Source: CAD feature listing. Evaluate the final solid. Frame: model axes, mm. Round coordinates to 2 decimals unless told otherwise and drop trailing zeros. Loops run counter-clockwise (first coordinate to the right, second up) from the corner with the lowest first, then second, coordinate; pieces in that order, holes last. Notation, with made-up numbers: (-22.75, -38) -> (6.25, -38) arc R35 cw to (6.25, -6) -> close; hole circle Ø9 at (-40, 11.25). An arc over 180 degrees is marked (long way). Write item = value, one per line.
from build123d import *

# Parameters (mm, degrees)
F1_DEPTH = 6.35
F2_R     = 2
F3_DEPTH = 20000
F4_R     = 7.5
F5_DEPTH = 55.3


with BuildPart() as f1:
    # F0 (on Top) → F1 (new body)
    with BuildSketch(Plane.XY):
        with BuildLine():
            ThreePointArc((86.6025406101, -49.9999995987), (96.5925826889, -25.8819042865), (100, 0))
            ThreePointArc((100, 0), (96.5925827815, 25.8819039408), (86.602540968, 49.9999989789))
            ThreePointArc((86.602540968, 49.9999989789), (50.0000005105, 86.6025400837), (0, 100))
            ThreePointArc((0, 100), (-50.0000005105, 86.6025400837), (-86.602540968, 49.9999989789))
            ThreePointArc((-86.602540968, 49.9999989789), (-100, 8.447e-07), (-86.6025418126, -49.9999975159))
            ThreePointArc((-86.6025418126, -49.9999975159), (-50.000001242, -86.6025396613), (0, -100))
            ThreePointArc((0, -100), (50.0000002007, -86.6025402626), (86.6025406101, -49.9999995987))
        make_face()
        with BuildLine():
            ThreePointArc((86.602540968, 49.9999989789), (96.5925827815, 25.8819039408), (100, 0))
            ThreePointArc((100, 0), (96.5925826889, -25.8819042865), (86.6025406101, -49.9999995987))
            Line((86.6025406101, -49.9999995987), (115.4700538379, 0))
            Line((115.4700538379, 0), (86.602540968, 49.9999989789))
        make_face()
        with BuildLine():
            ThreePointArc((0, 100), (50.0000005105, 86.6025400837), (86.602540968, 49.9999989789))
            Line((86.602540968, 49.9999989789), (57.735026919, 100))
            Line((57.735026919, 100), (0, 100))
        make_face()
        with BuildLine():
            Line((57.735026919, -100), (86.6025406101, -49.9999995987))
            ThreePointArc((86.6025406101, -49.9999995987), (50.0000002007, -86.6025402626), (0, -100))
            Line((0, -100), (57.735026919, -100))
        make_face()
        with BuildLine():
            ThreePointArc((-86.602540968, 49.9999989789), (-50.0000005105, 86.6025400837), (0, 100))
            Line((0, 100), (-57.735026919, 100))
            Line((-57.735026919, 100), (-86.602540968, 49.9999989789))
        make_face()
        with BuildLine():
            Line((-57.735026919, -100), (0, -100))
            ThreePointArc((0, -100), (-50.000001242, -86.6025396613), (-86.6025418126, -49.9999975159))
            Line((-86.6025418126, -49.9999975159), (-57.735026919, -100))
        make_face()
        with BuildLine():
            ThreePointArc((-86.6025418126, -49.9999975159), (-100, 8.447e-07), (-86.602540968, 49.9999989789))
            Line((-86.602540968, 49.9999989789), (-115.4700538379, 0))
            Line((-115.4700538379, 0), (-86.6025418126, -49.9999975159))
        make_face()
    extrude(amount=F1_DEPTH)

    # F2 (on Top) → F3 (cut)
    with BuildSketch(Plane.XY):
        with Locations((38.148275573, 95)):
            Circle(F2_R)
        with Locations((-38.148275573, 95)):
            Circle(F2_R)
        with Locations((-63.198275573, 80.5373757568)):
            Circle(F2_R)
        with Locations((-101.346551146, 14.4626242432)):
            Circle(F2_R)
        with Locations((-101.346551146, -14.4626242432)):
            Circle(F2_R)
        with Locations((-63.198275573, -80.5373757568)):
            Circle(F2_R)
        with Locations((-38.148275573, -95)):
            Circle(F2_R)
        with Locations((38.148275573, -95)):
            Circle(F2_R)
        with Locations((63.198275573, -80.5373757568)):
            Circle(F2_R)
        with Locations((101.346551146, -14.4626242432)):
            Circle(F2_R)
        with Locations((101.346551146, 14.4626242432)):
            Circle(F2_R)
        with Locations((63.198275573, 80.5373757568)):
            Circle(F2_R)
    extrude(amount=F3_DEPTH, mode=Mode.SUBTRACT)

    # F4 (on Top) → F5 (cut)
    with BuildSketch(Plane.XY):
        Circle(F4_R)
    extrude(amount=F5_DEPTH, mode=Mode.SUBTRACT)


solid = f1.part
1. Section query A-A (x = 0). Return the cut outline in (y, z).
Evaluation:
outline = (-100, 0) -> (-7.5, 0) -> (-7.5, 6.35) -> (-100, 6.35) -> close; (7.5, 0) -> (100, 0) -> (100, 6.35) -> (7.5, 6.35) -> close
2. Section query C-C (y = -67). Return the cut outline in (x, z), then the cut area to 3 significant figures.
Evaluation:
outline = (-76.79, 0) -> (76.79, 0) -> (76.79, 6.35) -> (-76.79, 6.35) -> close
area = 975 mm²
3. Section query D-D (x = -94.5). Return the cut outline in (y, z), then the cut area to 3 significant figures.
Evaluation:
outline = (-36.32, 0) -> (36.32, 0) -> (36.32, 6.35) -> (-36.32, 6.35) -> close
area = 461 mm²
4. Section query B-B (z = 3.5). Give the number of separate pieces and of enclosed holes in the cut face, then the cut area to 3 significant figures.
Evaluation:
separate_pieces = 1
enclosed_holes = 13
area = 34,300 mm²
5. Mould query, pull axis Y, two halves, no side actions, for faces 1 (the face through (-1, -100, 3)), 2 (the face through (1, 100, 3)), 3 (the face through (-7.493, 0.33, 3.131)). Classes: released by +Y, released by -Y, zero draft, split by the parting line, or undercut.
Evaluation:
face_1 = released by -Y
face_2 = released by +Y
face_3 = undercut
6. Contact query for a flat-ended pin moving along its axis: pin 1 Ø3 at (y, z) = (-72.5, 2) entering from +X. Output: stop coordinate, or through.
Evaluation:
pin_1 = 74.48
7. Line query: probe 1 along X at (y, z) = (0, 3.5); probe 2 along X at (y, z) = (95, 3); probe 3 along Y at (x, z) = (0, 1.5). Output: solid intervals per line, ascending. Write a range as from..to.
Evaluation:
probe_1 = -115.47..-7.5, 7.5..115.47
probe_2 = -60.62..-40.15, -36.15..36.15, 40.15..60.62
probe_3 = -100..-7.5, 7.5..100
